Geometry check sheet. Reference: drawing and pictorial views, mm from the part's lowest x, y, z. A direction names the side the tool comes from. Round coordinates to 2 decimals unless told otherwise and drop trailing zeros. Write each loop counter-clockwise with the first axis right and the second up, starting at its lowest first coordinate (ties: lowest second). Pieces come first, ordered by that corner, then holes. Notation, with made-up numbers: M 6.5,-20 L 12.5,-20 A19 cw 12.5,15 Z; hole C 79,37.25 d9. An arc over 180 degrees is marked long. Answer in a Markdown table with one row per item.
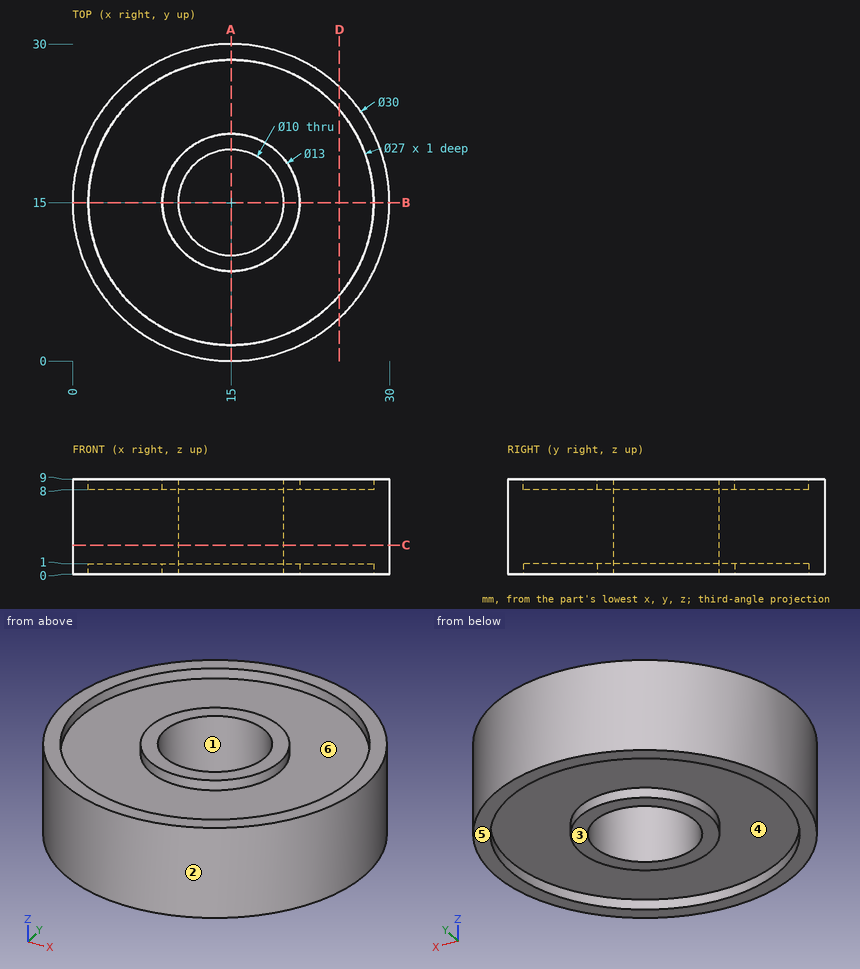
1. Access from +Z, -Z, +X, -X, +Y, -Y to the whole of each face (thin tool, end or side, straight path). Record for the marked faces 5 and 6.
Found:
| item | result |
|---|---|
| face 5 | -Z, +X, -X, +Y, -Y |
| face 6 | +Z |
2. Section check A-A, the plane x = 15. Record the cut outline in (y, z), and give its area (3 significant figures).
Found:
| item | result |
|---|---|
| outline | M 0,0 L 1.5,0 L 1.5,1 L 8.5,1 L 8.5,0 L 10,0 L 10,9 L 8.5,9 L 8.5,8 L 1.5,8 L 1.5,9 L 0,9 Z; M 20,0 L 21.5,0 L 21.5,1 L 28.5,1 L 28.5,0 L 30,0 L 30,9 L 28.5,9 L 28.5,8 L 21.5,8 L 21.5,9 L 20,9 Z |
| area | 152 mm2 |
3. Draft check along Y on the marked faces 1, 2, 3 and 4. Enter one of: +Y half, -Y half, draft (parallel to the pull), parting line (faces both ways), or undercut.
Found:
| item | result |
|---|---|
| face 1 | undercut |
| face 2 | parting line |
| face 3 | draft |
| face 4 | undercut |
4. Scan lines: L1, parallel to Y at x = 15, z = 3.25; L2, parallel to X at y = 19, z = 0.75; L3, parallel to Z at x = 27.5, y = 10. Record each from-to range of solid material in increasing order.
Found:
| item | result |
|---|---|
| L1 | y = 0 to 10, 20 to 30 |
| L2 | x = 0.54 to 2.11, 9.88 to 12, 18 to 20.12, 27.89 to 29.46 |
| L3 | z = 1 to 8 |
5. Go/stop test with flat-tipped pins: pin 1 (3 mm diameter, centred on x = 25.5, z = 6.5, fed in from -Y); pin 2 (2 mm diameter, centred on x = 19, z = 4, fed in from -Y); pin 3 (9 mm diameter, centred on x = 15, y = 15, fed in from -Z); pin 4 (1.5 mm diameter, centred on x = 8.5, y = 24, fed in from +Z). Record where each tip stops, or that it passes through.
Found:
| item | result |
|---|---|
| pin 1 | stops at y = 3 |
| pin 2 | stops at y = 0.3 |
| pin 3 | passes through |
| pin 4 | stops at z = 8 |
6. Section check C-C, the plane z = 2.75. Record the cut outline in (x, y), and give its area (3 significant figures).
Found:
| item | result |
|---|---|
| outline | C 15,15 d30; hole C 15,15 d10 |
| area | 628 mm2 |
7. Section check D-D, the plane x = 25.25. Record the cut outline in (y, z).
Found:
| item | result |
|---|---|
| outline | M 4.05,0 L 6.21,0 L 6.21,1 L 23.79,1 L 23.79,0 L 25.95,0 L 25.95,9 L 23.79,9 L 23.79,8 L 6.21,8 L 6.21,9 L 4.05,9 Z |
